Work out the finished part from the listing and answer in its coordinate system (mm). A direction names the side the tool comes from. Coordinates: 2 decimals unless noted, no trailing zeros. Order: outer loops, then holes, each group sorted by start corner. A loop starts at its lowest first (then second) coordinate and runs counter-clockwise, first axis right, second up. Notation, with made-up numbers: M -7,37.25 L 7,37.25 A22 ccw 7,70.25 Z; hole C -9,30.5 d5. An arc over 180 degrees is marked long. Answer in a Markdown table with one row per item. Add a question column.
Item 1: Flat-ended cylindrical pins translate along their axes: pin 1 Ø1.4 at (x, y) = (-7.92, -7.5) entering from -Z (3 decimals); pin 2 Ø4 at (x, z) = (29.5, 6.5) entering from +Y; pin 3 Ø4 at (x, z) = (35, 6) entering from -Y; pin 4 Ø3 at (y, z) = (22.5, 10) entering from +X. Find the tip coordinate at first contact, or state that the pin passes through.
Item 2: The part is cut by section B-B (z = 8). Write down the section's boundary in (x, y).
Item 3: The mould has two halves that part along X. Classify faces 5 (the face through (31.7, -9.41, 7.1)), 6 (the face through (25, 15, 7)), 7 (the face through (0, 25, 7)): released by +X, released by -X, zero draft, split by the parting line, or undercut.
Item 4: The part is cut by section C-C (y = -7.5). Write down the section's boundary in (x, z).
Item 5: Which of the six approach directions +Z, -Z, +X, -X, +Y, -Y give full straight-line access (tool end or side, diameter ignored) to faces 1 (the face through (25, -15, 7)), 2 (the face through (33, 13.434, 7)), 3 (the face through (-23, -16.899, 7)), 4 (the face through (-16.899, 23, 7))?
Item 6: Consider line 1 (Y direction, x = 30.9, z = 5.75); line 2 (X direction, y = 12, z = 4.25); line 3 (Y direction, x = 9.4, z = 9.5). Determine where each line is inside the solid, lowest interval first. Write a range as from..to.
Item 7: The part is cut by section A-A (x = 37.4). Write down the section's boundary in (y, z), then the cut area to 3 significant figures.
Autodesk Inventor part; units mm, degrees
ref_plane "YZ Plane" through (0, 0, 0) normal (1, 0, 0) x (0, 1, 0)
ref_plane "XZ Plane" through (0, 0, 0) normal (0, 1, 0) x (-1, 0, 0)
ref_plane "XY Plane" through (0, 0, 0) normal (0, 0, 1) x (1, 0, 0)
sketch "Sketch1" plane through (0, 0, 0) normal (0, 0, 1) x (1, 0, 0)
  line L0 (-37.8611, 0) -> (52.8619, 0) construction
  line L1 (0, -34.8609) -> (0, 34.8609) construction
  line L2 (0, 0) -> (13.4339, 13.4339) construction
  line L3 (0, 0) -> (18.9985, 0) construction
  line L4 (0, 24.9006) -> (16.8, 24.9006)
  line L5 (16.8, 24.9006) -> (16.8, 21.2406)
  line L6 (16.8, 21.2406) -> (19.0203, 19.0203)
  line L7 (24.9006, 0) -> (24.9006, 16.8)
  line L8 (24.9006, 16.8) -> (21.2406, 16.8)
  line L9 (21.2406, 16.8) -> (19.0203, 19.0203)
  line L10 (0, 0) -> (-13.4339, 13.4339) construction
  line L11 (0, 0) -> (-18.9985, 0) construction
  line L12 (0, 24.9006) -> (-16.8, 24.9006)
  line L13 (-16.8, 24.9006) -> (-16.8, 21.2406)
  line L14 (-16.8, 21.2406) -> (-19.0203, 19.0203)
  line L15 (-24.9006, 0) -> (-24.9006, 16.8)
  line L16 (-24.9006, 16.8) -> (-21.2406, 16.8)
  line L17 (-21.2406, 16.8) -> (-19.0203, 19.0203)
  line L18 (0, 0) -> (13.4339, -13.4339) construction
  line L19 (0, -24.9006) -> (16.8, -24.9006)
  line L20 (16.8, -24.9006) -> (16.8, -21.2406)
  line L21 (16.8, -21.2406) -> (19.0203, -19.0203)
  line L22 (24.9006, 0) -> (24.9006, -16.8)
  line L23 (24.9006, -16.8) -> (21.2406, -16.8)
  line L24 (21.2406, -16.8) -> (19.0203, -19.0203)
  line L25 (0, 0) -> (-13.4339, -13.4339) construction
  line L26 (0, -24.9006) -> (-16.8, -24.9006)
  line L27 (-16.8, -24.9006) -> (-16.8, -21.2406)
  line L28 (-16.8, -21.2406) -> (-19.0203, -19.0203)
  line L29 (-24.9006, 0) -> (-24.9006, -16.8)
  line L30 (-24.9006, -16.8) -> (-21.2406, -16.8)
  line L31 (-21.2406, -16.8) -> (-19.0203, -19.0203)
  circle A0 centre (37.4, 10.6752) radius 1
  circle A1 centre (30.9, -9.8248) radius 1
  line L32 (39.9015, 13.4339) -> (24.9006, 13.4339)
  line L33 (24.9006, 13.4339) -> (24.9006, -12.4218)
  line L34 (24.9006, -12.4218) -> (39.9015, -12.4218)
  line L35 (39.9015, -12.4218) -> (39.9015, 13.4339)
  dimension "d0" = 45
  dimension "d1" = 3.14
  dimension "d2" = 3.66
  dimension "d3" = 16.8
extrude "Thickness" add sketch "Sketch1" along normal blind 14 contours L4 L5 L6 L9 L8 L7 L22 L23 L24 L21 L20 L19 L26 L27 L28 L31 L30 L29 L15 L16 L17 L14 L13 L12 | L32 L35 L34 L22 L7 | A0 | A1
sketch "Sketch3" plane through (0, 0, 0) normal (0, 0, -1) x (-1, 0, 0)
  line L0 (-16.8, 24.9006) -> (16.8, 24.9006)
  line L1 (16.8, 24.9006) -> (16.8, 21.2406)
  line L2 (16.8, 21.2406) -> (21.2406, 16.8)
  line L3 (21.2406, 16.8) -> (24.9006, 16.8)
  line L4 (24.9006, 16.8) -> (24.9006, -16.8)
  line L5 (24.9006, -16.8) -> (21.2406, -16.8)
  line L6 (21.2406, -16.8) -> (16.8, -21.2406)
  line L7 (16.8, -21.2406) -> (16.8, -24.9006)
  line L8 (16.8, -24.9006) -> (-16.8, -24.9006)
  line L9 (-16.8, -24.9006) -> (-16.8, -21.2406)
  line L10 (-16.8, -21.2406) -> (-21.2406, -16.8)
  line L11 (-21.2406, -16.8) -> (-24.9006, -16.8)
  line L12 (-24.9006, -16.8) -> (-24.9006, -12.4218)
  line L13 (-24.9006, 16.8) -> (-21.2406, 16.8)
  line L14 (-21.2406, 16.8) -> (-16.8, 21.2406)
  line L15 (-16.8, 21.2406) -> (-16.8, 24.9006)
  line L16 (16.8994, 25) -> (-16.8994, 25)
  line L17 (-16.8994, 25) -> (-16.8994, 21.2818)
  line L18 (-16.8994, 21.2818) -> (-21.2818, 16.8994)
  line L19 (-21.2818, 16.8994) -> (-25, 16.8994)
  line L20 (-25, 16.8994) -> (-25, -16.8994)
  line L21 (-25, -16.8994) -> (-21.2818, -16.8994)
  line L22 (-21.2818, -16.8994) -> (-16.8994, -21.2818)
  line L23 (-16.8994, -21.2818) -> (-16.8994, -25)
  line L24 (-16.8994, -25) -> (16.8994, -25)
  line L25 (16.8994, -25) -> (16.8994, -21.2818)
  line L26 (16.8994, -21.2818) -> (21.2818, -16.8994)
  line L27 (21.2818, -16.8994) -> (25, -16.8994)
  line L28 (25, -16.8994) -> (25, 16.8994)
  line L29 (25, 16.8994) -> (21.2818, 16.8994)
  line L30 (21.2818, 16.8994) -> (16.8994, 21.2818)
  line L31 (16.8994, 21.2818) -> (16.8994, 25)
  line L32 (-39.9015, 13.4339) -> (-24.9006, 13.4339)
  line L33 (-24.9006, 13.4339) -> (-24.9006, 16.8)
  line L34 (-24.9006, -12.4218) -> (-39.9015, -12.4218)
  line L35 (-39.9015, -12.4218) -> (-39.9015, 13.4339)
  point P0 (0, 0)
  dimension "d22" = 50
extrude "Extrusion3" add sketch "Sketch3" against normal up to surface (14 mm away)
ref_plane "Work Plane1" through (0, -16.8994, 0) normal (-1, 0, 0) x (0, 0, 1)
ref_plane "Work Plane2" through (-16.8994, 0, 0) normal (0, -1, 0) x (1, 0, 0)
sketch "Sketch4" plane through (0, 0, 0) normal (0, 0, -1) x (-1, 0, 0)
  arc A0 (12.7755, -29.7) -> (13.7755, -30.7) centre (13.7755, -29.7) ccw
  line L0 (13.7755, -30.7) -> (16.92, -30.7)
  line L1 (16.92, -30.7) -> (16.92, -5)
  line L2 (16.92, -5) -> (7.3923, -5)
  arc A1 (7.3923, -5) -> (6.3923, -6) centre (7.3923, -6) ccw
  line L3 (6.3923, -6) -> (6.3923, -7.8624)
  arc A2 (5.3923, -8.8624) -> (6.3923, -7.8624) centre (5.3923, -7.8624) ccw
  line L4 (5.3923, -8.8624) -> (-13.08, -8.8624)
  line L5 (-13.08, -8.8624) -> (-13.08, -20.397)
  arc A3 (-14.08, -21.397) -> (-13.08, -20.397) centre (-14.08, -20.397) ccw
  line L6 (-14.08, -21.397) -> (-15.08, -21.397)
  arc A4 (-15.08, -21.397) -> (-16.08, -22.397) centre (-15.08, -22.397) ccw
  line L7 (-16.08, -22.397) -> (-16.08, -24.9624)
  arc A5 (-16.08, -24.9624) -> (-15.08, -25.9624) centre (-15.08, -24.9624) ccw
  line L8 (-15.08, -25.9624) -> (11.7755, -25.9624)
  arc A6 (12.7755, -26.9624) -> (11.7755, -25.9624) centre (11.7755, -26.9624) ccw
  line L9 (12.7755, -26.9624) -> (12.7755, -29.7)
  line L10 (4.42, -24) -> (-11.08, -24)
  line L11 (-11.08, -24) -> (-11.08, -10.5)
  line L12 (-11.08, -10.5) -> (4.42, -10.5)
  line L13 (4.42, -10.5) -> (4.42, -24)
  circle A7 centre (14.42, -28) radius 1
  circle A8 centre (7.92, -7.5) radius 1
  circle A9 centre (-13.58, -23) radius 1
  arc A10 (12.7755, 5.3) -> (13.7755, 4.3) centre (13.7755, 5.3) ccw
  line L14 (13.7755, 4.3) -> (16.92, 4.3)
  line L15 (16.92, 4.3) -> (16.92, 30)
  line L16 (16.92, 30) -> (7.3923, 30)
  arc A11 (7.3923, 30) -> (6.3923, 29) centre (7.3923, 29) ccw
  line L17 (6.3923, 29) -> (6.3923, 27.1376)
  arc A12 (5.3923, 26.1376) -> (6.3923, 27.1376) centre (5.3923, 27.1376) ccw
  line L18 (5.3923, 26.1376) -> (-13.08, 26.1376)
  line L19 (-13.08, 26.1376) -> (-13.08, 14.603)
  arc A13 (-14.08, 13.603) -> (-13.08, 14.603) centre (-14.08, 14.603) ccw
  line L20 (-14.08, 13.603) -> (-15.08, 13.603)
  arc A14 (-15.08, 13.603) -> (-16.08, 12.603) centre (-15.08, 12.603) ccw
  line L21 (-16.08, 12.603) -> (-16.08, 10.0376)
  arc A15 (-16.08, 10.0376) -> (-15.08, 9.0376) centre (-15.08, 10.0376) ccw
  line L22 (-15.08, 9.0376) -> (11.7755, 9.0376)
  arc A16 (12.7755, 8.0376) -> (11.7755, 9.0376) centre (11.7755, 8.0376) ccw
  line L23 (12.7755, 8.0376) -> (12.7755, 5.3)
  line L24 (4.42, 11) -> (-11.08, 11)
  line L25 (-11.08, 11) -> (-11.08, 24.5)
  line L26 (-11.08, 24.5) -> (4.42, 24.5)
  line L27 (4.42, 24.5) -> (4.42, 11)
  circle A17 centre (14.42, 7) radius 1
  circle A18 centre (7.92, 27.5) radius 1
  circle A19 centre (-13.58, 12) radius 1
  arc A20 (-35.7555, 12.3752) -> (-36.7555, 13.3752) centre (-36.7555, 12.3752) ccw
  line L28 (-36.7555, 13.3752) -> (-39.9, 13.3752)
  line L29 (-39.9, 13.3752) -> (-39.9, -12.3248)
  line L30 (-39.9, -12.3248) -> (-30.3723, -12.3248)
  arc A21 (-30.3723, -12.3248) -> (-29.3723, -11.3248) centre (-30.3723, -11.3248) ccw
  line L31 (-29.3723, -11.3248) -> (-29.3723, -9.4624)
  arc A22 (-28.3723, -8.4624) -> (-29.3723, -9.4624) centre (-28.3723, -9.4624) ccw
  line L32 (-28.3723, -8.4624) -> (-9.9, -8.4624)
  line L33 (-9.9, -8.4624) -> (-9.9, 3.0723)
  arc A23 (-8.9, 4.0723) -> (-9.9, 3.0723) centre (-8.9, 3.0723) ccw
  line L34 (-8.9, 4.0723) -> (-7.9, 4.0723)
  arc A24 (-7.9, 4.0723) -> (-6.9, 5.0723) centre (-7.9, 5.0723) ccw
  line L35 (-6.9, 5.0723) -> (-6.9, 7.6376)
  arc A25 (-6.9, 7.6376) -> (-7.9, 8.6376) centre (-7.9, 7.6376) ccw
  line L36 (-7.9, 8.6376) -> (-34.7555, 8.6376)
  arc A26 (-35.7555, 9.6376) -> (-34.7555, 8.6376) centre (-34.7555, 9.6376) ccw
  line L37 (-35.7555, 9.6376) -> (-35.7555, 12.3752)
  line L38 (-27.4, 6.6752) -> (-11.9, 6.6752)
  line L39 (-11.9, 6.6752) -> (-11.9, -6.8248)
  line L40 (-11.9, -6.8248) -> (-27.4, -6.8248)
  line L41 (-27.4, -6.8248) -> (-27.4, 6.6752)
  circle A27 centre (-37.4, 10.6752) radius 1
  circle A28 centre (-30.9, -9.8248) radius 1
  circle A29 centre (-9.4, 5.6752) radius 1
  point P0 (0, 0)
hole "Hole2" at (-7.92, -7.5, 0) at (-14.42, 7, 0) at (13.58, 12, 0) at (9.4, 5.6752, 0) at (30.9, -9.8248, 0) at (37.4, 10.6752, 0) direction (0, 0, 1) diameter 1.8 end through all
equation "\"Lens_diameter\" = 25.4"
properties part number "20_Cube_Insert_VCM_MirrorMount_KES400A"
Reply:
| question | item | result |
|---|---|---|
| 1 | pin 1 | passes through |
| 1 | pin 2 | stops at y = 13.43 |
| 1 | pin 3 | stops at y = -12.42 |
| 1 | pin 4 | stops at x = 17.18 |
| 2 | outline | M -25,-16.9 L -21.28,-16.9 L -16.9,-21.28 L -16.9,-25 L 16.9,-25 L 16.9,-21.28 L 21.28,-16.9 L 25,-16.9 L 25,-12.42 L 39.9,-12.42 L 39.9,13.43 L 25,13.43 L 25,16.9 L 21.28,16.9 L 16.9,21.28 L 16.9,25 L -16.9,25 L -16.9,21.28 L -21.28,16.9 L -25,16.9 Z; hole C -14.42,7 d1.8; hole C -7.92,-7.5 d1.8; hole C 9.4,5.68 d1.8; hole C 13.58,12 d1.8; hole C 30.9,-9.82 d1.8; hole C 37.4,10.68 d1.8 |
| 3 | face 5 | undercut |
| 3 | face 6 | released by +X |
| 3 | face 7 | zero draft |
| 4 | outline | M -25,0 L -8.82,0 L -8.82,14 L -25,14 Z; M -7.02,0 L 39.9,0 L 39.9,14 L -7.02,14 Z |
| 5 | face 1 | +Z, -Z, +X, -Y |
| 5 | face 2 | +Z, -Z, +X, +Y |
| 5 | face 3 | +Z, -Z, -X, -Y |
| 5 | face 4 | +Z, -Z, -X, +Y |
| 6 | line 1 | y = -12.42..-10.72, -8.92..13.43 |
| 6 | line 2 | x = -25..12.68, 14.48..39.9 |
| 6 | line 3 | y = -25..4.78, 6.58..25 |
| 7 | outline | M -12.42,0 L 9.78,0 L 9.78,14 L -12.42,14 Z; M 11.58,0 L 13.43,0 L 13.43,14 L 11.58,14 Z |
| 7 | area | 337 mm2 |
